Autodesk Inventor part; units mm, degrees
ref_plane "YZ Plane" through (0, 0, 0) normal (1, 0, 0) x (0, 1, 0)
ref_plane "XZ Plane" through (0, 0, 0) normal (0, 1, 0) x (-1, 0, 0)
ref_plane "XY Plane" through (0, 0, 0) normal (0, 0, 1) x (1, 0, 0)
sketch "Sketch1" plane through (0, 0, 0) normal (0, 1, 0) x (-1, 0, 0)
  circle A0 centre (0, 0) radius 4
  circle A1 centre (0, 0) radius 2.6
  dimension "d0" = 8
  dimension "d1" = 5.2
extrude "Extrusion1" add sketch "Sketch1" along normal blind 5
sketch "Sketch2" plane through (0, 5, 0) normal (0, 1, 0) x (1, 0, 0)
  circle A0 centre (0, 0) radius 4
  circle A1 centre (0, 0) radius 1.5
  circle A2 centre (0, 0) radius 4
  dimension "d4" = 3
  dimension "d5" = 8
extrude "Extrusion2" add sketch "Sketch2" along normal blind 50
sketch "Sketch3" plane through (0, 55, 0) normal (0, 1, 0) x (1, 0, 0)
  circle A0 centre (0, 0) radius 2.5
  dimension "d8" = 5
extrude "Extrusion3" cut sketch "Sketch3" against normal blind 5
properties part number "MountScrew_test"
Read the model definition and answer for the solid it produces. Units are mm, in the model's axes. A direction names the side the tool comes from. Round coordinates to 2 decimals unless told otherwise and drop trailing zeros. Write each loop counter-clockwise with the first axis right and the second up, starting at its lowest first coordinate (ties: lowest second). Pieces come first, ordered by that corner, then holes. Notation, with made-up numbers: M 25,-23.5 L 71,-23.5 A29 cw 71,1.5 Z; hole C 17,75 d4. An arc over 180 degrees is marked long. Use a Markdown table: item, result.
1) A tool of negligible diameter and unlimited length cuts with its end or side. For faces 4 (the cylindrical face through (0.338, 2.465, -2.578)), 5 (the cylindrical face through (-0.54, 52.54, 2.44)), 6 (the flat face through (-3, 0, 0)), from which of +Z, -Z, +X, -X, +Y, -Y can it reach the whole face along a straight path? Write none if from no direction.
Answers follow:
| item | result |
|---|---|
| face 4 | -Y |
| face 5 | +Y |
| face 6 | +Z, -Z, +X, -X, -Y |
2) The part is cut by section B-B (z = -2). Write down the section's boundary in (x, y), plus the area to 3 significant figures.
Answers follow:
| item | result |
|---|---|
| outline | M -3.46,0 L -1.66,0 L -1.66,5 L 1.66,5 L 1.66,0 L 3.46,0 L 3.46,55 L 1.5,55 L 1.5,50 L -1.5,50 L -1.5,55 L -3.46,55 Z |
| area | 349 mm2 |
3) Straight lines are drawn through the part: line 1 along X through (y, z) = (51.85, 0); line 2 along X through (y, z) = (34.5, 0); line 3 along Z through (x, y) = (0, 2.1). For each, find the intervals that lie inside material, in ascending order. Write a range as [from, to].
Answers follow:
| item | result |
|---|---|
| line 1 | x = [-4, -2.5], [2.5, 4] |
| line 2 | x = [-4, -1.5], [1.5, 4] |
| line 3 | z = [-4, -2.6], [2.6, 4] |
4) For a pull along Z with two mould halves and no side action, classify faces 1 (the flat face through (2, 5, 0)), 2 (the cylindrical face through (0, 27, 4)), 3 (the flat face through (2, 55, -2)) as pulls with the +Z half, pulls with the -Z half, needs draft (parallel to the pull), parting line crosses it, or undercut.
Answers follow:
| item | result |
|---|---|
| face 1 | undercut |
| face 2 | parting line crosses it |
| face 3 | needs draft |
5) The part is cut by section C-C (y = 30). Write down the section's boundary in (x, z), plus the area to 3 significant figures.
Answers follow:
| item | result |
|---|---|
| outline | C 0,0 d8; hole C 0,0 d3 |
| area | 43.2 mm2 |
6) Flat-ended cylindrical pins translate along their axes: pin 1 (3 mm diameter, centred on x = -2, z = -2, fed in from -Y); pin 2 (4 mm diameter, centred on x = 0, z = 0, fed in from -Y); pin 3 (1 mm diameter, centred on y = 29.5, z = -2, fed in from -X); pin 4 (1 mm diameter, centred on y = 44, z = -1.5, fed in from +X). Find the tip coordinate at first contact, or state that the pin passes through.
Answers follow:
| item | result |
|---|---|
| pin 1 | stops at y = 0 |
| pin 2 | stops at y = 5 |
| pin 3 | stops at x = -3.71 |
| pin 4 | stops at x = 3.87 |
